Answer from the drawing. Dimensions are ordinates in mm from the lowest x, y and z of the part. A direction names the side the tool comes from. Coordinates: 2 decimals unless noted, no trailing zeros. Order: outer loops, then holes, each group sorted by start corner. A loop starts at its lowest first (then second) coordinate and runs counter-clockwise, first axis right, second up.
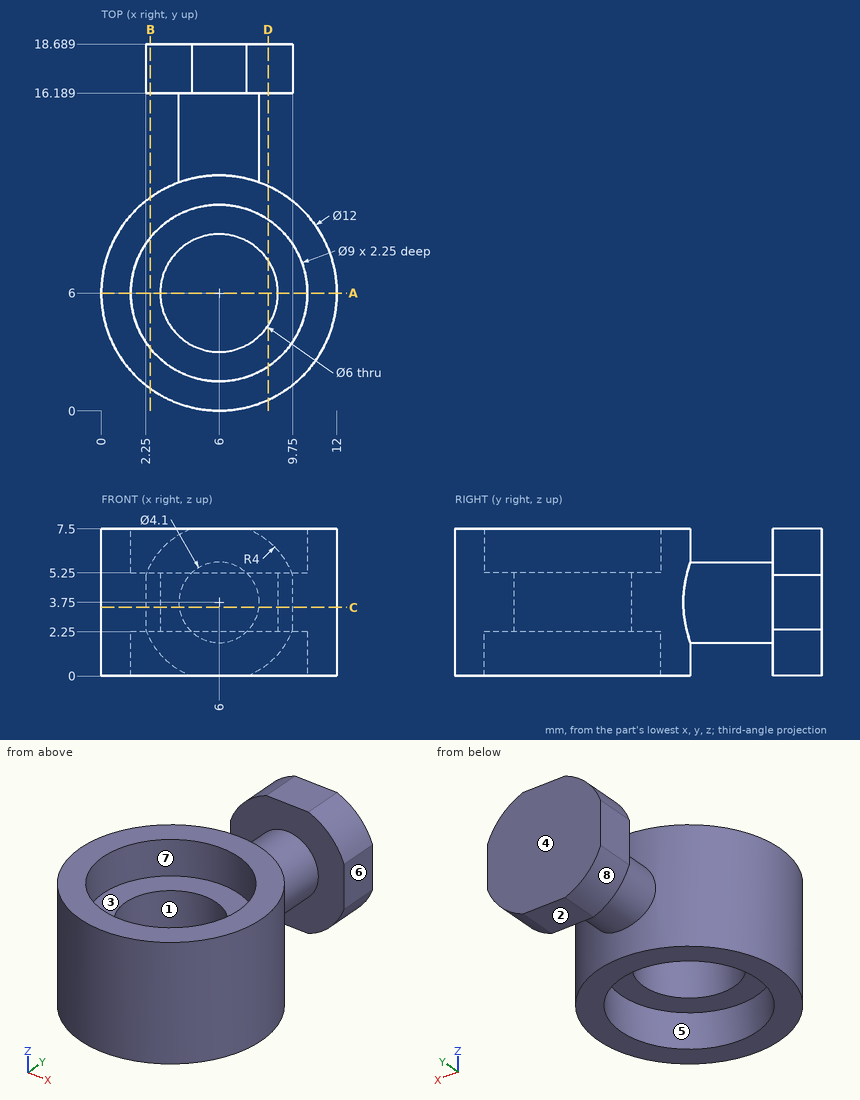
1. Consider probe 1 along Y at (x, z) = (6, 0.6); probe 2 along Y at (x, z) = (8, 2); probe 3 along X at (y, z) = (16.75, 3). Determine where each line is inside the solid, lowest interval first.
2. The part is cut by section D-D (x = 8.5). Determine the outline of the cut face in (y, z).
3. The part is cut by section C-C (z = 3.5). Determine the outline of the cut face in (x, y).
4. The mould has two halves that part along Y. Classify the marked faces 1, 2, 3 and 4: released by +Y, released by -Y, zero draft, split by the parting line, or undercut.
5. The part is cut by section A-A (y = 6). Determine the outline of the cut face in (x, z), plus the area to 3 significant figures.
6. The part is cut by section B-B (x = 2.5). Determine the outline of the cut face in (y, z), plus the area to 3 significant figures.
7. For the marked faces 5, 6, 7 and 8, determine the directions among +Z, -Z, +X, -X, +Y, -Y from which every point of the face is accessible in a straight line to the end or side of a thin tool.
8. Flat-ended cylindrical pins translate along their axes: pin 1 (0.8 mm diameter, centred on y = 18, z = 3.5, fed in from +X); pin 2 (7 mm diameter, centred on x = 6, y = 6, fed in from -Z); pin 3 (3 mm diameter, centred on y = 17, z = 3, fed in from -X). Find the tip coordinate at first contact, or state that the pin passes through.
Worked out:
1. probe 1: y = 0 to 1.5, 10.5 to 12, 16.19 to 18.69
1. probe 2: y = 0.34 to 1.97, 10.03 to 11.66, 16.19 to 18.69
1. probe 3: x = 2.25 to 9.75
2. outline: (0.55, 0) - (2.26, 0) - (2.26, 2.25) - (4.34, 2.25) - (4.34, 5.25) - (2.26, 5.25) - (2.26, 7.5) - (0.55, 7.5) - close; (7.66, 2.25) - (9.74, 2.25) - (9.74, 0) - (11.45, 0) - (11.45, 7.5) - (9.74, 7.5) - (9.74, 5.25) - (7.66, 5.25) - close; (16.19, 0.63) - (18.69, 0.63) - (18.69, 6.87) - (16.19, 6.87) - close
3. outline: (2.25, 16.19) - (3.97, 16.19) - (3.97, 11.64) arc R6 ccw (long way) to (8.03, 11.64) - (8.03, 16.19) - (9.75, 16.19) - (9.75, 18.69) - (2.25, 18.69) - close; hole circle Ø6 at (6, 6)
4. face 1: undercut
4. face 2: zero draft
4. face 3: undercut
4. face 4: released by +Y
5. outline: (0, 0) - (1.5, 0) - (1.5, 2.25) - (3, 2.25) - (3, 5.25) - (1.5, 5.25) - (1.5, 7.5) - (0, 7.5) - close; (9, 2.25) - (10.5, 2.25) - (10.5, 0) - (12, 0) - (12, 7.5) - (10.5, 7.5) - (10.5, 5.25) - (9, 5.25) - close
5. area: 31.5 mm2
6. outline: (1.13, 0) - (3.17, 0) - (3.17, 2.25) - (8.83, 2.25) - (8.83, 0) - (10.87, 0) - (10.87, 7.5) - (8.83, 7.5) - (8.83, 5.25) - (3.17, 5.25) - (3.17, 7.5) - (1.13, 7.5) - close; (16.19, 1.81) - (18.69, 1.81) - (18.69, 5.69) - (16.19, 5.69) - close
6. area: 57.3 mm2
7. face 5: -Z
7. face 6: +Z, -Z, +X, +Y
7. face 7: +Z
7. face 8: -Z, -X, +Y
8. pin 1: stops at x = 9.75
8. pin 2: stops at z = 2.25
8. pin 3: stops at x = 2.25
